The model under review builds one solid part; all positions refer to its coordinate system, in mm. A direction names the side the tool comes from. Coordinates: 2 decimals unless noted, no trailing zeros. Order: outer loops, then holes, each group sorted by start corner. A loop starts at its lowest first (then second) coordinate and runs counter-clockwise, first axis right, second up. Notation, with made-up numbers: (-5, 72.5) - (1, 72.5) arc R26 cw to (1, 108.5) - close; hole circle Ø7 at (80, 44). An arc over 180 degrees is marked (long way). Answer in a Markdown table with one row per item.
```python
from build123d import *

# Parameters (mm, degrees)
F0_R          = 0.5
F1_DEPTH      = 10
F0_R_2        = 1
F2_DEPTH      = 0.25
F3_R          = 0.12
F5_DEPTH      = 5
F5_DEPTH_BACK = 5
F7_DEPTH      = 25
F7_DEPTH_BACK = 25


with BuildPart() as f1:
    # F0 (on Right) → F1 (new body)
    with BuildSketch(Plane.YZ):
        Circle(F0_R)
    extrude(amount=F1_DEPTH)

    # F0 (on Right) → F2 (join)
    with BuildSketch(Plane.YZ):
        Circle(F0_R_2)
        Circle(F0_R, mode=Mode.SUBTRACT)
        Circle(F0_R)
    extrude(amount=-F2_DEPTH)

    # F3
    f3_edges = [f1.edges().sort_by_distance(p)[0] for p in [
        (-0.25, -1, 0),
    ]]
    fillet(f3_edges, radius=F3_R)

    # F4 (on Front) → F5 (cut, two sides)
    with BuildSketch(Plane.XZ) as f5_sk:
        Polygon((8.994769305, 0.8649917436), (9.9934805185, 0), (9.1212727129, -0.79286861), (10.6126805767, -1.0325592011), (10.7525009662, 0.9182563517), align=None)
    extrude(amount=F5_DEPTH, mode=Mode.SUBTRACT)
    extrude(f5_sk.sketch, amount=-F5_DEPTH_BACK, mode=Mode.SUBTRACT)

    # F6 (on Top) → F7 (cut, two sides)
    with BuildSketch(Plane.XY) as f7_sk:
        Polygon((10.3356074542, 0.6147447275), (9.5979655161, 0.6147447275), (9.9958730862, 0), (9.5723690465, -0.6511143292), (10.3356074542, -0.6511143292), align=None)
    extrude(amount=F7_DEPTH, mode=Mode.SUBTRACT)
    extrude(f7_sk.sketch, amount=-F7_DEPTH_BACK, mode=Mode.SUBTRACT)


solid = f1.part
```
Item 1: Tool access review of faces 1 (the face through (-0.25, 0, 0)), 2 (the face through (4.79, -0.108, -0.488)): name each direction out of +Z, -Z, +X, -X, +Y, -Y from which nothing blocks a thin tool from reaching the whole face with its end or side.
Check values:
| item | result |
|---|---|
| face 1 | +Z, -Z, -X, +Y, -Y |
| face 2 | +X |
Item 2: We need section A-A, the plane x = 7.75. Write out the cut boundary in (y, z).
Check values:
| item | result |
|---|---|
| outline | circle Ø1 at (0, 0) |
Item 3: To check wall thickness, follow line 1 (Z direction, x = 8, y = 0.25); line 2 (Z direction, x = 0.75, y = 0); line 3 (X direction, y = -0.4, z = -0.6). State the ranges of each line that lie inside material, in increasing order. Write a range as from..to.
Check values:
| item | result |
|---|---|
| line 1 | -0.43..0.43 |
| line 2 | -0.5..0.5 |
| line 3 | -0.25..0 |
